```python
from build123d import *

# Parameters (mm, degrees)
SKETCH1_W           = 12
SKETCH1_H           = 12
BOSS_EXTRUDE1_DEPTH = 3
SKETCH2_W           = 0.6
SKETCH2_H           = 0.5
BOSS_EXTRUDE2_DEPTH = 2.5


with BuildPart() as part:
    # Sketch1 → Boss-Extrude1 (new body)
    with BuildSketch(Plane(origin=(0, 0, 0), x_dir=(1, 0, 0), z_dir=(0, 1, 0))):
        Rectangle(SKETCH1_W, SKETCH1_H)
    extrude(amount=BOSS_EXTRUDE1_DEPTH)

    # Sketch2 → Boss-Extrude2 (add, symmetric)
    with BuildSketch(Plane.XY.offset(6)):
        with Locations((4.7, -0.25)):
            Rectangle(SKETCH2_W, SKETCH2_H)
        with Locations((-4.7, -0.25)):
            Rectangle(SKETCH2_W, SKETCH2_H)
    boss_extrude2 = extrude(amount=BOSS_EXTRUDE2_DEPTH, both=True)

    # Mirror1: Boss-Extrude2 across plane
    add(boss_extrude2.mirror(Plane.XY))


solid = part.part
```
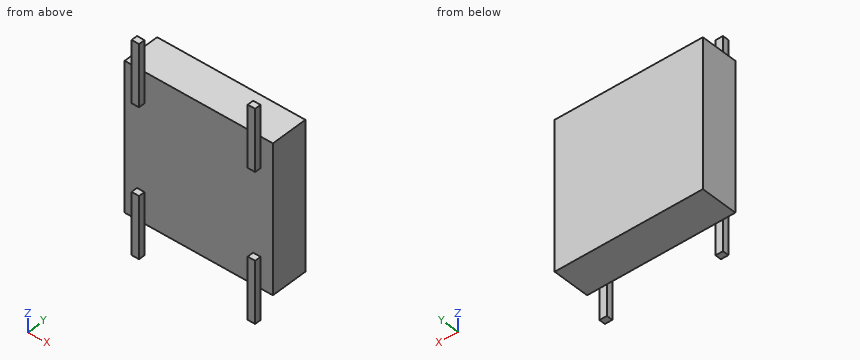
For this review, take the finished solid that the model builds, in its own axes (mm). Round coordinates to 2 decimals unless told otherwise and drop trailing zeros. Write each loop counter-clockwise with the first axis right and the second up, starting at its lowest first coordinate (ties: lowest second). Pieces come first, ordered by that corner, then holes. Notation, with made-up numbers: (-29, 38) -> (-1, 38) arc R8 cw to (-1, 46) -> close; hole circle Ø9 at (-35, 56.25). An arc over 180 degrees is marked (long way). One line per question, with ' | ' between items. Start each with the question number.
1) Add section B-B (y = 2.8). Write out the cut boundary in (x, z).
2) Wall thickness on line 1 along X through (y, z) = (-0.2, -8); line 2 along Z through (x, y) = (-1.75, 1.1); line 3 along Y through (x, z) = (3.5, 1.75): over which ranges is each line inside the solid? List them lowest first.
3) For pin 1 Ø0.5 at (x, z) = (-4.5, -7.5) entering from +Y; pin 2 Ø1.5 at (x, y) = (1, 1.5) entering from +Z; pin 3 Ø0.6 at (y, z) = (-0.5, -5) entering from -X, all flat-tipped, find the tip position at first contact; note any pin that passes through.
4) Add section A-A (z = 6.5). Write out the cut boundary in (x, y), and give its area (3 significant figures).
5) Add section C-C (z = 2.5). Write out the cut boundary in (x, y), and give its area (3 significant figures).
Reported:
1) outline: (-6, -6) -> (6, -6) -> (6, 6) -> (-6, 6) -> close
2) line 1: x = -5 to -4.4, 4.4 to 5 | line 2: z = -6 to 6 | line 3: y = 0 to 3
3) pin 1: stops at y = 0 | pin 2: stops at z = 6 | pin 3: stops at x = -5
4) outline: (-5, -0.5) -> (-4.4, -0.5) -> (-4.4, 0) -> (-5, 0) -> close; (4.4, -0.5) -> (5, -0.5) -> (5, 0) -> (4.4, 0) -> close | area: 0.600 mm²
5) outline: (-6, 0) -> (6, 0) -> (6, 3) -> (-6, 3) -> close | area: 36.0 mm²
